Autodesk Inventor part; units mm, degrees
ref_plane "YZ Plane" through (0, 0, 0) normal (1, 0, 0) x (0, 1, 0)
ref_plane "XZ Plane" through (0, 0, 0) normal (0, 1, 0) x (-1, 0, 0)
ref_plane "XY Plane" through (0, 0, 0) normal (0, 0, 1) x (1, 0, 0)
sketch "Náčrt1" plane through (0, 0, 0) normal (0, 1, 0) x (-1, 0, 0)
  line L0 (49.75, -24.25) -> (49.75, 44.75)
  line L1 (49.75, 44.75) -> (-49.75, 44.75)
  line L2 (-49.75, 44.75) -> (-49.75, -24.25)
  line L3 (-49.75, -24.25) -> (-27, -24.25)
  line L4 (-27, -24.25) -> (-27, -44.75)
  line L5 (-27, -44.75) -> (27, -44.75)
  line L6 (27, -44.75) -> (27, -24.25)
  line L7 (27, -24.25) -> (49.75, -24.25)
  line L8 (49.75, -44.75) -> (0, 0) construction
  line L9 (0, 0) -> (-49.75, -44.75) construction
  line L10 (49.75, 44.75) -> (0, 0) construction
  line L11 (-49.75, 44.75) -> (0, 0) construction
  dimension "d0" = 99.5
  dimension "d1" = 89.5
  dimension "d2" = 20.5
  dimension "d3" = 54
extrude "Vysunutí1" add sketch "Náčrt1" along normal blind 5
sketch "Náčrt2" plane through (0, 5, 0) normal (0, 1, 0) x (1, 0, 0)
  circle A0 centre (0, -35.833) radius 5
  circle A1 centre (41.463, -35.833) radius 5
  circle A2 centre (-41.136, -35.833) radius 5
  circle A3 centre (0, 40.875) radius 5
  line L0 (49.75, -44.75) -> (49.75, 24.25)
  line L1 (-49.75, 24.25) -> (-49.75, -44.75)
  line L2 (-49.75, -44.75) -> (49.75, -44.75)
  line L3 (27, 44.75) -> (-27, 44.75)
  line L4 (-5, 40.875) -> (-5, 44.75)
  line L5 (5, 40.875) -> (5, 44.75)
  point P0 (0, 0)
  point P1 (3.1598, 44.75)
  point P2 (-3.1598, 44.75)
  dimension "d6" = 10
  dimension "d7" = 8.287
  dimension "d8" = 8.614
  dimension "d9" = 8.917
  dimension "d10" = 3.875
extrude "Vysunutí2" cut sketch "Náčrt2" against normal through all
sketch "Náčrt3" plane through (49.75, 0, 44.75) normal (1, 0, 0) x (0, 0, -1)
  line L0 (0, 0) -> (69, 0)
  line L1 (0, 0) -> (1.3397, 5)
  line L2 (69, 5) -> (0, 5)
  line L3 (0, 0) -> (0, 5)
  point P0 (44.75, 0)
  dimension "d13" = 75
extrude "Vysunutí3" cut sketch "Náčrt3" against normal through all
sketch "Náčrt4" plane through (0, 0, 0) normal (0, -1, 0) x (1, 0, 0)
  line L0 (49.75, -24.25) -> (27, -24.25)
  line L1 (49.75, 44.75) -> (49.75, -24.25)
  line L2 (-49.75, -24.25) -> (-49.75, 44.75)
  line L3 (-27, -44.75) -> (-27, -24.25)
  line L4 (27, -24.25) -> (27, -44.75)
  point P0 (0, 0)
  point P1 (42.25, -13.5)
  point P2 (-42.25, -13.5)
  point P3 (42.25, 24)
  point P4 (-42.25, 24)
  point P5 (22, -29.1875)
  point P6 (-22, -29.1875)
  dimension "d16" = 10.75
  dimension "d17" = 7.5
  dimension "d18" = 7.5
  dimension "d19" = 37.5
  dimension "d27" = 5
  dimension "d28" = 5
  dimension "d29" = 4.9375
hole "Díra1" at (-42.25, 0, -13.5) at (-42.25, 0, 24) at (42.25, 0, 24) at (42.25, 0, -13.5) at (22, 0, -29.1875) at (-22, 0, -29.1875) direction (0, 1, 0) diameter 3.5 end through all countersink diameter 7 countersink angle 90
properties part number "plech"
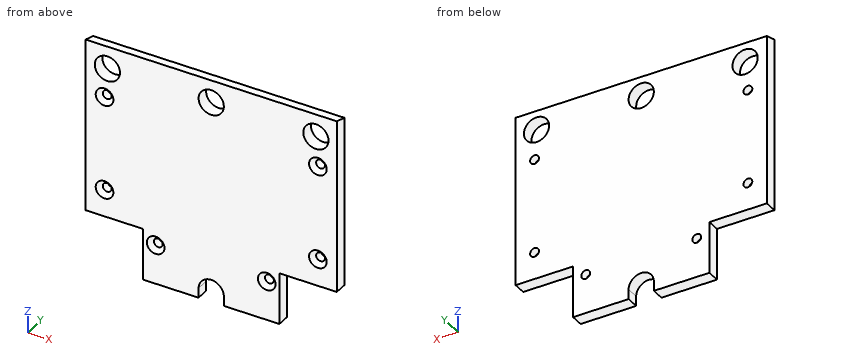
Verification items for the finished model (mm, model axes). Give positions to 0.01 mm unless a question says otherwise; leave off trailing zeros. Loops run counter-clockwise (first coordinate to the right, second up) from the corner with the lowest first, then second, coordinate; pieces in that order, holes last. Notation, with made-up numbers: M -1.75,32.5 L 55.25,32.5 A15 ccw 55.25,43.5 Z; hole C -27,-0.75 d9. An arc over 180 degrees is marked long. One line per question, with ' | ' between items.
Item 1: Thickness scan on line 1 (X direction, y = 4.3, z = 24); line 2 (X direction, y = 0.55, z = -14); line 3 (Z direction, x = -42.25, y = 3.45). Record the ranges inside material, lowest first. Write a range as [from, to].
Completed:
line 1: x = [-49.75, -44], [-40.5, 40.5], [44, 49.75] | line 2: x = [-49.75, -45.16], [-39.34, 39.34], [45.16, 49.75] | line 3: z = [-24.25, -15.25], [-11.75, 22.25], [25.75, 30.96], [40.71, 43.83]
Item 2: Section check A-A, the plane z = -13.5. Record the cut outline in (x, y), plus the area to 3 significant figures.
Completed:
outline: M -49.75,0 L -45.75,0 L -44,1.75 L -44,5 L -49.75,5 Z; M -40.5,1.75 L -38.75,0 L 38.75,0 L 40.5,1.75 L 40.5,5 L -40.5,5 Z; M 44,1.75 L 45.75,0 L 49.75,0 L 49.75,5 L 44,5 Z | area: 456 mm^2
Item 3: Section check B-B, the plane x = 22. Record the cut outline in (y, z), plus the area to 3 significant figures.
Completed:
outline: M 0,-44.75 L 5,-44.75 L 5,-30.94 L 1.75,-30.94 L 0,-32.69 Z; M 0,-25.69 L 1.75,-27.44 L 5,-27.44 L 5,43.41 L 0,44.75 Z | area: 424 mm^2
Item 4: Depth check by flat-ended pin: P1, Ø4, axis at x = -20, z = -4.5, coming from the -Y side; P2, Ø2, axis at x = 28, y = 2, coming from the +Z side; P3, Ø1.5, axis at x = 40.5, y = 2, coming from the -Z side; P4, Ø3, axis at x = -42.25, z = 24, coming from the +Y side. Enter the tip coordinate at first touch or a pass-through.
Completed:
P1: stops at y = 0 | P2: stops at z = 44.48 | P3: stops at z = -24.25 | P4: passes through
Item 5: Section check D-D, the plane y = 0.95. State how many separate pieces and enclosed holes the cut face has, plus the area to 3 significant figures.
Completed:
separate pieces: 1 | enclosed holes: 9 | area: 7,510 mm^2
Item 6: Section check C-C, the plane z = -38. Record the cut outline in (x, y).
Completed:
outline: M -27,0 L -4.09,0 L -4.09,5 L -27,5 Z; M 4.09,0 L 27,0 L 27,5 L 4.09,5 Z
